Autodesk Inventor part; units mm, degrees
ref_plane "YZ Plane" through (0, 0, 0) normal (1, 0, 0) x (0, 1, 0)
ref_plane "XZ Plane" through (0, 0, 0) normal (0, 1, 0) x (-1, 0, 0)
ref_plane "XY Plane" through (0, 0, 0) normal (0, 0, 1) x (1, 0, 0)
sketch "Sketch1" plane through (0, 0, 0) normal (0, 1, 0) x (-1, 0, 0)
  line L0 (7.8238, 10.3217) -> (-12.1762, 10.3217)
  line L1 (-12.1762, 10.3217) -> (-12.1762, -12.6783)
  line L2 (-12.1762, -12.6783) -> (7.8238, -12.6783)
  line L3 (7.8238, -12.6783) -> (7.8238, 10.3217)
  line L4 (7.8238, 10.3217) -> (-12.1762, 10.3217)
  line L5 (-12.1762, 10.3217) -> (-12.1762, 7.3217)
  line L6 (-12.1762, 7.3217) -> (7.8238, 7.3217)
  line L7 (7.8238, 7.3217) -> (7.8238, 10.3217)
  line L8 (7.8238, -12.6783) -> (-12.1762, -12.6783)
  line L9 (-12.1762, -12.6783) -> (-12.1762, -9.6783)
  line L10 (-12.1762, -9.6783) -> (7.8238, -9.6783)
  line L11 (7.8238, -9.6783) -> (7.8238, -12.6783)
  point P0 (0, 0)
  dimension "d0" = 23
  dimension "d1" = 20
  dimension "d2" = 3
  dimension "d3" = 3
extrude "Extrusion1" add sketch "Sketch1" along normal blind 28 contours L3 L6 L1 L0 | L3 L2 L1 L10
sketch "Sketch2" plane through (-7.8238, 0, 10.3217) normal (0, 0, 1) x (1, 0, 0)
  circle A0 centre (10, 10) radius 2.75
  circle A1 centre (10, 23) radius 2.75
  line L0 (0, 0) -> (20, 0)
  line L1 (0, 28) -> (20, 28)
  line L2 (0, 0) -> (0, 28)
  point P0 (7.8238, 0)
  dimension "d6" = 5.5
  dimension "d7" = 5.5
  dimension "d8" = 10
  dimension "d9" = 5
  dimension "d10" = 10
extrude "Extrusion2" cut sketch "Sketch2" against normal through all
sketch "Sketch3" plane through (12.1762, 0, -9.6783) normal (1, 0, 0) x (0, 0, -1)
  line L0 (3, 28) -> (-20, 28)
  line L1 (-20, 28) -> (-20, -20)
  line L2 (-20, -20) -> (3, -20)
  line L3 (3, -20) -> (3, 28)
  point P0 (-9.6783, 0)
  dimension "d13" = 48
extrude "Extrusion3" add sketch "Sketch3" along normal blind 3
sketch "Sketch4" plane through (15.1762, 0, -9.6783) normal (1, 0, 0) x (0, 0, -1)
  circle A0 centre (-15, -10) radius 2.75
  line L0 (-20, -20) -> (3, -20)
  line L1 (-20, 28) -> (-20, -20)
  circle A1 centre (-2, -10) radius 2.75
  line L2 (3, -20) -> (3, 28)
  point P0 (-9.6783, 0)
  dimension "d16" = 5.5
  dimension "d17" = 10
  dimension "d18" = 5
  dimension "d21" = 13
  dimension "d26" = 5
extrude "Extrusion4" cut sketch "Sketch4" against normal blind 3
fillet "Fillet1" radius 0.5 3 edges at (12.1762, -10, 10.3217) (15.1762, 4, 10.3217) (-7.8238, 14, 10.3217)
fillet "Fillet1" radius 0.5 17 edges at (-7.8238, 14, 7.3217) (-7.8238, 14, -9.6783) (-7.8238, 14, -12.6783) (2.1762, 28, 7.3217) (12.1762, 28, -1.1783) (2.1762, 28, -9.6783) (3.6762, 28, -12.6783) (15.1762, 28, -1.1783) (3.6762, 28, 10.3217) (12.1762, -10, -12.6783) (15.1762, 4, -12.6783) (12.1762, -20, -1.1783) (15.1762, -20, -1.1783) (2.1762, 0, 7.3217) (2.1762, 0, 10.3217) (2.1762, 0, -9.6783) (2.1762, 0, -12.6783)
fillet "Fillet2" radius 0.5 10 edges at (12.3227, 27.8536, 7.4682) (12.1762, 0.1464, 7.4682) (12.1762, 0, 8.8217) (12.3227, 0.1464, 10.1753) (12.1762, 14, 7.3217) (12.3227, 27.8536, -9.8247) (12.1762, 0.1464, -9.8247) (12.1762, 0, -11.1783) (12.3227, 0.1464, -12.5318) (12.1762, 14, -9.6783)
properties part number "bottom printhead screwplate_250221"
Input: part model. Units: mm. Frame: model coordinates. A direction names the side the tool comes from. Round coordinates to 2 decimals unless told otherwise and drop trailing zeros. Loops run counter-clockwise (first coordinate to the right, second up) from the corner with the lowest first, then second, coordinate; pieces in that order, holes last. Notation, with made-up numbers: M 13.5,-24 L 40.5,-24 A4 ccw 40.5,-19 Z; hole C 74.25,28 d10. An arc over 180 degrees is marked long. Answer as CSV lines item,"result". Start each with the question number.
(1) Line query: line 1 (Z direction, x = 6, y = 20.5); line 2 (Y direction, x = 1.5, z = 9); line 3 (X direction, y = -6, z = -3.5). Output: solid intervals per line, ascending. Write a range as [from, to].
(2) Draft query along Z for faces 4 (the flat face through (2, 14, 7.322)), 5 (the flat face through (4, 15, 10.322)), 6 (the cylindrical face through (1.818, 25.727, 8.843)). Return one class per face: released by +Z, released by -Z, zero draft, split by the parting line, or undercut.
(3) Reachability of faces 1 (the flat face through (2, 14, -9.678)), 2 (the flat face through (2, 0, -11)), 3 (the cylindrical face through (1.818, 12.727, -11.157)) from +Z, -Z, +X, -X, +Y, -Y: full face, straight path, thin tool, end or side. Return the list, or none.
(4) First-contact query: pin 1 (6 mm diameter, centred on y = 4.5, z = -0.5, fed in from -X); pin 2 (5 mm diameter, centred on x = 2.5, z = 5.5, fed in from -Y). Flat tips, straight axial feed; report the tip coordinate or a pass-through.
(5) Section D-D, the plane x = 1.75. State how many separate pieces and enclosed holes the cut face has, plus the area to 3 significant figures.
(6) Section B-B, the plane x = -2.25. Output: boundary loops of the cut face in (y, z).
(7) Section A-A, the plane y = -10. Output: boundary loops of the cut face in (x, z), plus the area to 3 significant figures.
(8) Section C-C, the plane z = 8.75. Output: boundary loops of the cut face in (x, y).
Values found:
1,line 1,"z = [-12.68, -9.68], [7.32, 10.32]"
1,line 2,"y = [0, 7.33], [12.67, 20.33], [25.67, 28]"
1,line 3,"x = [12.18, 15.18]"
2,face 4,"undercut"
2,face 5,"released by +Z"
2,face 6,"zero draft"
3,face 1,"-X, +Y, -Y"
3,face 2,"+Z, -Z, -X, -Y"
3,face 3,"+Z, -Z"
4,pin 1,"stops at x = 12.18"
4,pin 2,"stops at y = 0"
5,separate pieces,"6"
5,enclosed holes,"0"
5,area,"102 mm²"
6,outline,"M 0,-12.18 A0.5 ccw 0.5,-12.68 L 27.5,-12.68 A0.5 ccw 28,-12.18 L 28,-10.18 A0.5 ccw 27.5,-9.68 L 0.5,-9.68 A0.5 ccw 0,-10.18 Z; M 0,7.82 A0.5 ccw 0.5,7.32 L 27.5,7.32 A0.5 ccw 28,7.82 L 28,9.82 A0.5 ccw 27.5,10.32 L 0.5,10.32 A0.5 ccw 0,9.82 Z"
7,outline,"M 12.18,-12.18 A0.5 ccw 12.68,-12.68 L 14.68,-12.68 A0.5 ccw 15.18,-12.18 L 15.18,-10.43 L 12.18,-10.43 Z; M 12.18,-4.93 L 15.18,-4.93 L 15.18,2.57 L 12.18,2.57 Z; M 12.18,8.07 L 15.18,8.07 L 15.18,9.82 A0.5 ccw 14.68,10.32 L 12.68,10.32 A0.5 ccw 12.18,9.82 Z"
7,area,"35.8 mm²"
8,outline,"M -7.82,0 L 11.68,0 A0.5 cw 12.18,-0.5 L 12.18,-19.5 A0.5 ccw 12.68,-20 L 14.68,-20 A0.5 ccw 15.18,-19.5 L 15.18,27.5 A0.5 ccw 14.68,28 L -7.82,28 Z; hole C 2.18,10 d5.5; hole C 2.18,23 d5.5"
